Job drawing, mm, ordinate dimensions from the low corner. One solid piece. Round coordinates to 2 decimals unless told otherwise and drop trailing zeros. Loops run counter-clockwise (first coordinate to the right, second up) from the corner with the lowest first, then second, coordinate; pieces in that order, holes last. Notation, with made-up numbers: M 19.5,-37.75 L 72.5,-37.75 A12 ccw 72.5,-24.75 Z; hole C 63,82.25 d11. An arc over 180 degrees is marked long. Use a Markdown table: item, result. Add a question column.
(1) Flat gauge pins, fed straight in: P1, Ø1.5, axis at y = 9.5, z = 34, coming from the -X side; P2, Ø3, axis at y = 15.5, z = 7.5, coming from the -X side; P3, Ø3, axis at x = 54.5, y = 15.5, coming from the -Z side; P4, Ø3, axis at y = 15.5, z = 20, coming from the -X side. Where does each tip first touch, or does it go through?
(2) Band-saw the part on C-C, the plane x = 56. Write the cut outline in (y, z).
(3) Band-saw the part on D-D, the plane z = 19. Write the cut outline in (x, y).
(4) Band-saw the part on B-B, the plane z = 41.5. Write the cut outline in (x, y).
(5) Band-saw the part on A-A, the plane y = 16.25. Write the cut outline in (x, z), and give its area (3 significant figures).
(6) Wall check: L1, parallel to Y at x = 30, z = 7.5; L2, parallel to Z at x = 51.5, y = 17.5; L3, parallel to X at y = 15, z = 40. Give the ranges that are in metal, low to high.
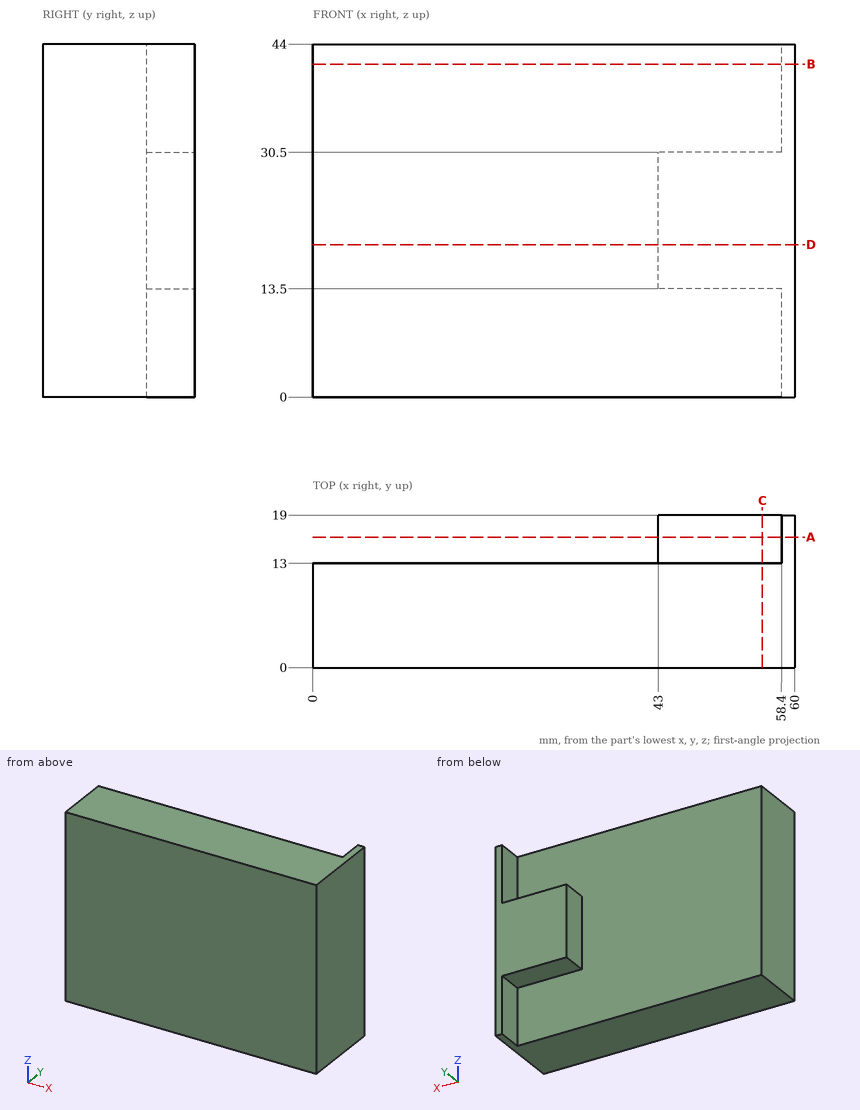
Return value:
| question | item | result |
|---|---|---|
| 1 | P1 | x = 0 |
| 1 | P2 | x = 58.4 |
| 1 | P3 | z = 13.5 |
| 1 | P4 | x = 43 |
| 2 | outline | M 0,0 L 13,0 L 13,13.5 L 19,13.5 L 19,30.5 L 13,30.5 L 13,44 L 0,44 Z |
| 3 | outline | M 0,0 L 60,0 L 60,19 L 43,19 L 43,13 L 0,13 Z |
| 4 | outline | M 0,0 L 60,0 L 60,19 L 58.4,19 L 58.4,13 L 0,13 Z |
| 5 | outline | M 43,13.5 L 58.4,13.5 L 58.4,0 L 60,0 L 60,44 L 58.4,44 L 58.4,30.5 L 43,30.5 Z |
| 5 | area | 332 mm^2 |
| 6 | L1 | 0 to 13 |
| 6 | L2 | 13.5 to 30.5 |
| 6 | L3 | 58.4 to 60 |
